Design review of the part built by this model. Coordinates are the model's own, in mm. Face numbers are marked on the shaded views. A direction names the side the tool comes from. Coordinates: 2 decimals unless noted, no trailing zeros. Order: outer loops, then holes, each group sorted by start corner. A loop starts at its lowest first (then second) coordinate and runs counter-clockwise, first axis right, second up. Notation, with made-up numbers: M 67,-15.5 L 123,-15.5 A22 cw 123,20.5 Z; hole C 64.25,49.25 d10. An arc over 180 degrees is marked long. Answer as a JSON object with one key per item and string values.
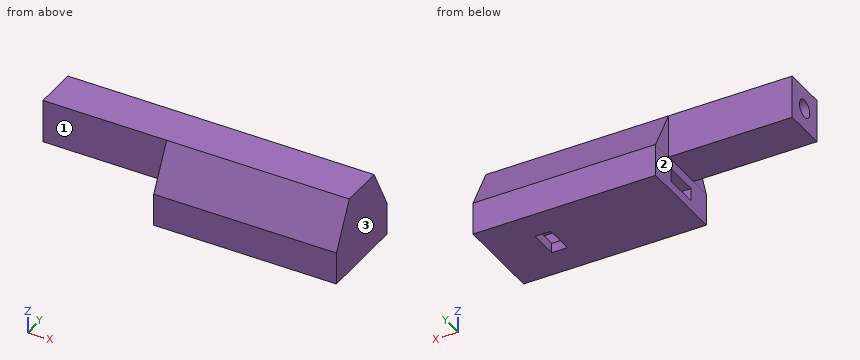
from build123d import *

# Parameters (mm, degrees)
F0_W      = 84.2419564724
F0_H      = 40.8445894718
F0_W_2    = 75
F0_H_2    = 16
F1_DEPTH  = 7.5
F2_W      = 16.3
F2_H      = 6
F3_DEPTH  = 73.5
F4_W      = 57.0175424218
F4_H      = 20
F4_W_2    = 84.2419564724
F5_DEPTH  = 20
F6_R      = 4.1
F7_DEPTH  = 134.3
F9_DEPTH  = 84.23
F10_W     = 7.2
F10_H     = 13.4
F11_DEPTH = 31.8


with BuildPart() as f1:
    # F0 (on Top) → F1 (new body, symmetric)
    with BuildSketch(Plane.XY):
        Rectangle(F0_W, F0_H)
        Rectangle(F0_W_2, F0_H_2, mode=Mode.SUBTRACT)
        Rectangle(F0_W_2, F0_H_2)
    extrude(amount=F1_DEPTH, both=True)

    # F2 (on face) → F3 (cut)
    with BuildSketch(Plane(origin=(-42.1209782362, 0, 0), x_dir=(0, -1, 0), z_dir=(-1, 0, 0))):
        Rectangle(F2_W, F2_H)
    extrude(amount=-F3_DEPTH, mode=Mode.SUBTRACT)

    # F4 (on face) → F5 (join)
    with BuildSketch(Plane.XY.offset(7.5)):
        with Locations((-70.6297494471, 0)):
            Rectangle(F4_W, F4_H)
        Rectangle(F4_W_2, F4_H)
    extrude(amount=F5_DEPTH)

    # F6 (on face) → F7 (cut)
    with BuildSketch(Plane(origin=(-99.138520658, 0, 0), x_dir=(0, -1, 0), z_dir=(-1, 0, 0))):
        with Locations((0, 17.5)):
            Circle(F6_R)
    extrude(amount=-F7_DEPTH, mode=Mode.SUBTRACT)

    # F8 (on face) → F9 (join)
    with BuildSketch(Plane.YZ.offset(42.1209782362)):
        Polygon((-10, 7.5), (-10, 27.5), (-20.4222947359, 7.5), align=None)
        Polygon((20.4222947359, 7.5), (10, 27.5), (10, 7.5), align=None)
    extrude(amount=-F9_DEPTH)

    # F10 (on face) → F11 (cut)
    with BuildSketch(Plane(origin=(0, 0, -7.5), x_dir=(1, 0, 0), z_dir=(0, 0, -1))):
        with Locations((17.7071348711, 0)):
            Rectangle(F10_W, F10_H)
    extrude(amount=-F11_DEPTH, mode=Mode.SUBTRACT)


solid = f1.part
1) Insertion check: pin 1 Ø7.5 at (y, z) = (-8, 1) entering from -X; pin 2 Ø1 at (x, z) = (-40.5, 18) entering from -Y; pin 3 Ø3.5 at (x, z) = (19.5, 17) entering from -Y. Each pin has a flat end and moves straight along its axis. Give the tip position at first contact, or say it passes through.
Taken from the geometry:
{"pin 1": "stops at x = -42.12", "pin 2": "stops at y = -15.21", "pin 3": "stops at y = -16.38"}
2) Add section B-B (x = -53). State the section outline as (y, z) points, and give its area (3 significant figures).
Taken from the geometry:
{"outline": "M -10,7.5 L 10,7.5 L 10,27.5 L -10,27.5 Z; hole C 0,17.5 d8.2", "area": "347 mm2"}
3) Add section C-C (x = -3.5). State the section outline as (y, z) points.
Taken from the geometry:
{"outline": "M -20.42,-7.5 L 20.42,-7.5 L 20.42,7.5 L 10,27.5 L -10,27.5 L -20.42,7.5 Z; hole M -8.15,-3 L 8.15,-3 L 8.15,3 L -8.15,3 Z; hole C 0,17.5 d8.2"}
4) Tool access review of the marked faces 1, 2 and 3: name each direction out of +Z, -Z, +X, -X, +Y, -Y from which nothing blocks a thin tool from reaching the whole face with its end or side.
Taken from the geometry:
{"face 1": "+Z, -Z, -X, -Y", "face 2": "-Z, -X, +Y, -Y", "face 3": "+Z, -Z, +X, +Y, -Y"}
5) Add section D-D (z = 17.5). State the section outline as (x, y) points, and give its area (3 significant figures).
Taken from the geometry:
{"outline": "M -99.14,-10 L -42.11,-10 L -42.11,-15.21 L 42.12,-15.21 L 42.12,15.21 L -42.11,15.21 L -42.11,10 L -99.14,10 L -99.14,4.1 L 14.11,4.1 L 14.11,6.7 L 21.31,6.7 L 21.31,4.1 L 35.16,4.1 L 35.16,-4.1 L 21.31,-4.1 L 21.31,-6.7 L 14.11,-6.7 L 14.11,-4.1 L -99.14,-4.1 Z", "area": "2,560 mm2"}
6) To check wall thickness, follow L1, parallel to Z at x = 31, y = 0; L2, parallel to Y at x = -71, z = 17; L3, parallel to Z at x = 10, y = 6. State the ranges of each line that lie inside material, in increasing order.
Taken from the geometry:
{"L1": "z = -7.5 to -3, 3 to 13.4, 21.6 to 27.5", "L2": "y = -10 to -4.07, 4.07 to 10", "L3": "z = -7.5 to -3, 3 to 27.5"}
7) Add section A-A (y = 0). State the section outline as (x, z) points.
Taken from the geometry:
{"outline": "M -99.14,7.5 L -42.12,7.5 L -42.12,3 L 14.11,3 L 14.11,13.4 L -99.14,13.4 Z; M -99.14,21.6 L 14.11,21.6 L 14.11,24.3 L 21.31,24.3 L 21.31,21.6 L 35.16,21.6 L 35.16,13.4 L 21.31,13.4 L 21.31,3 L 31.38,3 L 31.38,-3 L 21.31,-3 L 21.31,-7.5 L 42.12,-7.5 L 42.12,27.5 L -99.14,27.5 Z; M -42.12,-7.5 L 14.11,-7.5 L 14.11,-3 L -42.12,-3 Z"}
